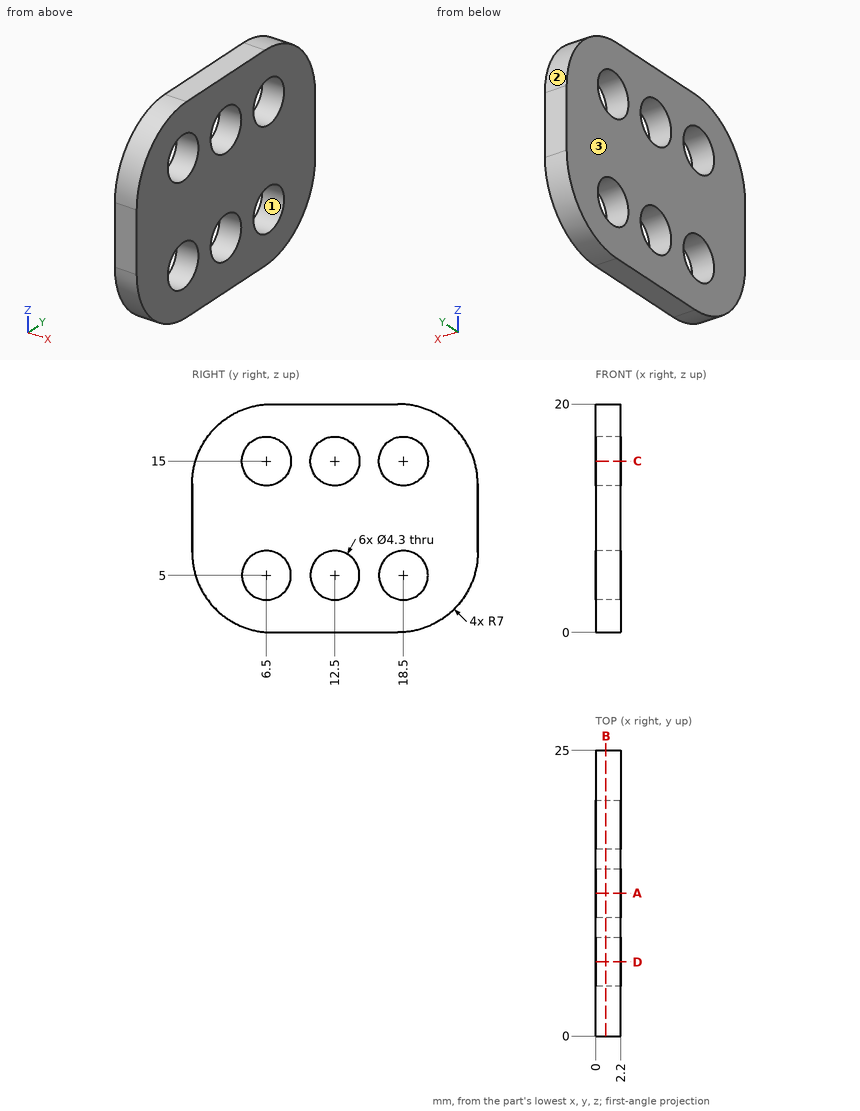
The drawing under review shows one solid part. Ordinate dimensions are in mm from its lowest x, y, z. Round coordinates to 2 decimals unless told otherwise and drop trailing zeros. Write each loop counter-clockwise with the first axis right and the second up, starting at its lowest first coordinate (ties: lowest second). Pieces come first, ordered by that corner, then holes. Notation, with made-up numbers: M -22.5,35.25 L 31.5,35.25 A19 ccw 31.5,50.25 Z; hole C -2,50.5 d9. An arc over 180 degrees is marked long. One line per item, written item: value. Start each with the question number.
(1) We need section C-C (z = 15). Give the boundary of the cut face in (x, y), and give its area (3 significant figures).
(2) The part is to be moulded in two halves that separate along Z. For the marked faces 1, 2 and 3, say which applies: released by +Z, released by -Z, zero draft, split by the parting line, or undercut.
(3) We need section B-B (x = 0.9). Give the boundary of the cut face in (y, z).
(4) We need section D-D (y = 6.5). Give the boundary of the cut face in (x, z).
(5) We need section A-A (y = 12.5). Give the boundary of the cut face in (x, z).
(6) Wall thickness on line 1 (Z direction, x = 2, y = 13.25); line 2 (Z direction, x = 0.6, y = 6.5); line 3 (Y direction, x = 1.5, z = 14.5): over which ranges is each line inside the solid? List them lowest first.
Result:
1. outline: M 0,0.29 L 2.2,0.29 L 2.2,4.35 L 0,4.35 Z; M 0,8.65 L 2.2,8.65 L 2.2,10.35 L 0,10.35 Z; M 0,14.65 L 2.2,14.65 L 2.2,16.35 L 0,16.35 Z; M 0,20.65 L 2.2,20.65 L 2.2,24.71 L 0,24.71 Z
1. area: 25.3 mm²
2. face 1: undercut
2. face 2: released by +Z
2. face 3: zero draft
3. outline: M 0,7 A7 ccw 7,0 L 18,0 A7 ccw 25,7 L 25,13 A7 ccw 18,20 L 7,20 A7 ccw 0,13 Z; hole C 6.5,5 d4.3; hole C 6.5,15 d4.3; hole C 12.5,5 d4.3; hole C 12.5,15 d4.3; hole C 18.5,5 d4.3; hole C 18.5,15 d4.3
4. outline: M 0,0.02 L 2.2,0.02 L 2.2,2.85 L 0,2.85 Z; M 0,7.15 L 2.2,7.15 L 2.2,12.85 L 0,12.85 Z; M 0,17.15 L 2.2,17.15 L 2.2,19.98 L 0,19.98 Z
5. outline: M 0,0 L 2.2,0 L 2.2,2.85 L 0,2.85 Z; M 0,7.15 L 2.2,7.15 L 2.2,12.85 L 0,12.85 Z; M 0,17.15 L 2.2,17.15 L 2.2,20 L 0,20 Z
6. line 1: 0 to 2.99, 7.01 to 12.99, 17.01 to 20
6. line 2: 0.02 to 2.85, 7.15 to 12.85, 17.15 to 19.98
6. line 3: 0.16 to 4.41, 8.59 to 10.41, 14.59 to 16.41, 20.59 to 24.84
